Geometry: final body of the model. Coordinates: model frame, mm. Face numbers are marked on the shaded views. A direction names the side the tool comes from. Give positions to 0.01 mm unless a question says otherwise; leave off trailing zeros. Write each loop counter-clockwise with the first axis right and the second up, starting at its lowest first coordinate (ties: lowest second). Pieces come first, ordered by that corner, then holes.
Q1. Line query: line 1 (X direction, y = 14, z = 11); line 2 (X direction, y = 10, z = 10.25); line 3 (Y direction, x = 18, z = 24). Output: solid intervals per line, ascending.
Q2. Section D-D (y = -14). Return the cut outline in (x, z) (3 decimals), plus the area to 3 significant figures.
Q3. Pin query (flat end, axial travel): pin 1 Ø10.5 at (x, y) = (-29.5, -7.5) entering from +Z; pin 2 Ø5 at (x, y) = (0, 15.5) entering from +Z; pin 3 Ø5.5 at (y, z) = (8.5, 13) entering from -X; pin 4 Ø5.5 at (y, z) = (5, 16.5) entering from +X. Return the tip coordinate at first contact, or that it passes through.
Q4. Mould query, pull axis X, two halves, no side actions, for the marked faces 6, 7, 8 and 9. Classes: +X half, -X half, draft (parallel to the pull), parting line (faces both ways), or undercut.
Q5. Section A-A (y = 13.5). Return the cut outline in (x, z).
Q6. Reachability of the marked faces 1, 2, 3, 4 and 5 from +Z, -Z, +X, -X, +Y, -Y: full face, straight path, thin tool, end or side. Return the list, or none.
Q7. Section C-C (x = -22). Return the cut outline in (y, z), plus the area to 3 significant figures.
from build123d import *

# Parameters (mm, degrees)
F0_W      = 76.2
F0_H      = 38.1
F1_DEPTH  = 25.4
F2_W      = 50.8
F2_H      = 6.35
F3_DEPTH  = 19.05
F4_W      = 6.35
F4_H      = 38.1
F5_DEPTH  = 19.05
F7_DEPTH  = 25.4
F8_R      = 3.81
F9_W      = 6.985
F9_H      = 19.05
F9_W_2    = 6.9872894436
F10_DEPTH = 19.05
F11_R     = 6.98499


# Not quite as in the source:
# - a fillet or chamfer is up to 0.001 mm smaller than in the source, because OpenCascade refuses the exact size
# - a feature of the source that left no trace in its solid (it failed there, or was rolled back) is left out


with BuildPart() as f1:
    # F0 (on Top) → F1 (new body)
    with BuildSketch(Plane.XY):
        Rectangle(F0_W, F0_H)
    extrude(amount=F1_DEPTH)

    # F2 (on face) → F3 (cut)
    with BuildSketch(Plane.XY.offset(25.4)):
        with Locations((0, 15.875)):
            Rectangle(F2_W, F2_H)
    extrude(amount=-F3_DEPTH, mode=Mode.SUBTRACT)

    # F4 (on face) → F5 (cut)
    with BuildSketch(Plane.XY.offset(25.4)):
        with Locations((-34.925, 0)):
            Rectangle(F4_W, F4_H)
        with Locations((34.925, 0)):
            Rectangle(F4_W, F4_H)
    extrude(amount=-F5_DEPTH, mode=Mode.SUBTRACT)

    # F6 (on face) → F7 (cut)
    with BuildSketch(Plane.XY.offset(25.4)):
        with BuildLine():
            Line((-12.7, -19.05), (12.7, -19.05))
            ThreePointArc((12.7, -19.05), (0, -6.35), (-12.7, -19.05))
        make_face()
    extrude(amount=-F7_DEPTH, mode=Mode.SUBTRACT)

    # F8
    f8_edges = [f1.edges().sort_by_distance(p)[0] for p in [
        (38.1, -19.05, 3.175),
        (-38.1, -19.05, 3.175),
    ]]
    fillet(f8_edges, radius=F8_R)

    # F9 (on face) → F10 (cut)
    with BuildSketch(Plane.XY.offset(25.4)):
        with Locations((-28.2575, -9.525)):
            Rectangle(F9_W, F9_H)
        with Locations((28.2563552782, -9.525)):
            Rectangle(F9_W_2, F9_H)
    extrude(amount=-F10_DEPTH, mode=Mode.SUBTRACT)

    # F11 (radius 6.985 in the source; OpenCascade refuses exactly that, so slightly less here)
    f11_edges = [f1.edges().sort_by_distance(p)[0] for p in [
        (24.762711, 0, 15.875),
        (-24.765, 0, 15.875),
    ]]
    fillet(f11_edges, radius=F11_R)


solid = f1.part
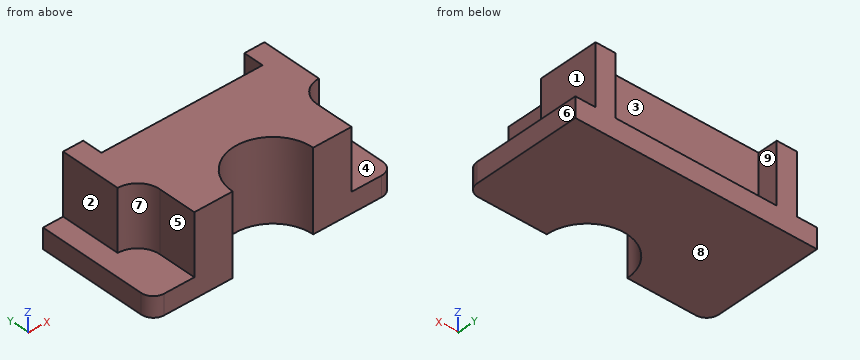
Computed:
1. line 1: x = -31.75 to -25.4, 25.4 to 31.75
1. line 2: x = -31.75 to 31.75
1. line 3: y = -19.05 to 12.7
2. outline: (-38.1, 0) - (-11.653, 0) - (-11.653, 25.4) - (-24.765, 25.4) - (-24.765, 6.35) - (-38.1, 6.35) - close; (11.653, 0) - (38.1, 0) - (38.1, 6.35) - (24.763, 6.35) - (24.763, 25.4) - (11.653, 25.4) - close
2. area: 835 mm2
3. pin 1: stops at z = 25.4
3. pin 2: stops at z = 6.35
3. pin 3: stops at x = -31.75
3. pin 4: stops at x = 31.75
4. face 6: +X half
4. face 7: -X half
4. face 8: draft
4. face 9: undercut
5. outline: (-38.1, 0) - (38.1, 0) - (38.1, 6.35) - (31.75, 6.35) - (31.75, 25.4) - (25.4, 25.4) - (25.4, 6.35) - (-25.4, 6.35) - (-25.4, 25.4) - (-31.75, 25.4) - (-31.75, 6.35) - (-38.1, 6.35) - close
6. face 1: +Z, +X, +Y, -Y
6. face 2: +Z, -X, +Y, -Y
6. face 3: +Z, +Y
6. face 4: +Z, +X, -Y
6. face 5: +Z, -X, -Y
7. outline: (-19.05, 0) - (19.05, 0) - (19.05, 6.35) - (12.7, 6.35) - (12.7, 25.4) - (-19.05, 25.4) - close
7. area: 847 mm2
